For this review, take the finished solid that the model builds, in its own axes (mm). A direction names the side the tool comes from. Coordinates: 2 decimals unless noted, no trailing zeros. Loops run counter-clockwise (first coordinate to the right, second up) from the corner with the lowest first, then second, coordinate; pieces in that order, holes last. Notation, with made-up numbers: (-14.5, -29) -> (-9.5, -29) arc R6 ccw to (-9.5, -25) -> close; hole circle Ø2 at (32.25, 19.5). An arc over 180 degrees is marked (long way). One line per item, written item: value.
from build123d import *

# Parameters (mm, degrees)
F1_DEPTH  = 44.45
F9_DEPTH  = 9.525
F10_DEPTH = 9.525
F12_DEPTH = 2.38125
F13_R     = 11.7475
F13_R_2   = 10.7315
F14_DEPTH = 7.9375
F15_DEPTH = 10.31875


with BuildPart() as f1:
    # F0 (on Top) → F1 (new body)
    with BuildSketch(Plane.XY):
        with BuildLine():
            ThreePointArc((-4.572, 0), (0, 4.572), (4.572, 0))
            Line((4.572, 0), (7.747, 0))
            ThreePointArc((7.747, 0), (5.951410253, 4.9595085442), (1.397, 7.62))
            ThreePointArc((1.397, 7.62), (0, 7.747), (-1.397, 7.62))
            ThreePointArc((-1.397, 7.62), (-5.951410253, 4.9595085442), (-7.747, 0))
            Line((-7.747, 0), (-4.572, 0))
        make_face()
        with BuildLine():
            ThreePointArc((-1.397, 7.62), (0, 7.747), (1.397, 7.62))
            Line((1.397, 7.62), (1.397, 19.3802))
            ThreePointArc((1.397, 19.3802), (0, 19.1615406713), (-1.397, 19.3802))
            Line((-1.397, 19.3802), (-1.397, 7.62))
        make_face()
        with BuildLine():
            ThreePointArc((-1.397, 19.3802), (0, 19.1615406713), (1.397, 19.3802))
            ThreePointArc((1.397, 19.3802), (3.6939320514, 21.0394638349), (4.572, 23.7335406713))
            ThreePointArc((4.572, 23.7335406713), (-2.6940768363, 27.4274727226), (-1.397, 19.3802))
        make_face()
    extrude(amount=F1_DEPTH)

    # F6 (on offset) → F9 (cut)
    with BuildSketch(Plane.XY.offset(28.575)):
        with BuildLine():
            ThreePointArc((4.1557772601, 1.7640375299), (0, -1.016), (-4.1557772601, 1.7640375299))
            Line((-4.1557772601, 1.7640375299), (-7.6070004234, 1.7640375299))
            ThreePointArc((-7.6070004234, 1.7640375299), (0, -4.318), (7.6070004234, 1.7640375299))
            Line((7.6070004234, 1.7640375299), (4.1557772601, 1.7640375299))
        make_face()
        with BuildLine():
            ThreePointArc((-4.1557772601, 1.7640375299), (-0.8747878771, 7.8904367738), (4.4961791045, 3.4801791045))
            ThreePointArc((4.4961791045, 3.4801791045), (4.4102576693, 2.6053912274), (4.1557772601, 1.7640375299))
            Line((4.1557772601, 1.7640375299), (7.6070004234, 1.7640375299))
            ThreePointArc((7.6070004234, 1.7640375299), (7.750237064, 2.6168003938), (7.7981791045, 3.4801791045))
            ThreePointArc((7.7981791045, 3.4801791045), (-0.8633787106, 11.2304161684), (-7.6070004234, 1.7640375299))
            Line((-7.6070004234, 1.7640375299), (-4.1557772601, 1.7640375299))
        make_face()
        with BuildLine():
            ThreePointArc((7.6070004234, 1.7640375299), (0, -4.318), (-7.6070004234, 1.7640375299))
            Line((-7.6070004234, 1.7640375299), (-8.4216929972, 1.7640375299))
            Line((-8.4216929972, 1.7640375299), (-8.4216929972, -6.3198274001))
            Line((-8.4216929972, -6.3198274001), (11.7628639564, -6.3198274001))
            Line((11.7628639564, -6.3198274001), (11.7628639564, 1.7640375299))
            Line((11.7628639564, 1.7640375299), (7.6070004234, 1.7640375299))
        make_face()
    extrude(amount=F9_DEPTH, mode=Mode.SUBTRACT)

    # F8 (on offset) → F10 (cut)
    with BuildSketch(Plane.XY.offset(15.875)):
        with BuildLine():
            ThreePointArc((4.179462045, 1.8225532258), (0, -1.016), (-4.179462045, 1.8225532258))
            Line((-4.179462045, 1.8225532258), (-7.6199654718, 1.8225532258))
            ThreePointArc((-7.6199654718, 1.8225532258), (0, -4.318), (7.6199654718, 1.8225532258))
            Line((7.6199654718, 1.8225532258), (4.179462045, 1.8225532258))
        make_face()
        with BuildLine():
            ThreePointArc((-4.179462045, 1.8225532258), (-0.8438058499, 7.8964692022), (4.4961791045, 3.4801791045))
            ThreePointArc((4.4961791045, 3.4801791045), (4.4162900977, 2.6363732546), (4.179462045, 1.8225532258))
            Line((4.179462045, 1.8225532258), (7.6199654718, 1.8225532258))
            ThreePointArc((7.6199654718, 1.8225532258), (7.7534976902, 2.6465899292), (7.7981791045, 3.4801791045))
            ThreePointArc((7.7981791045, 3.4801791045), (-0.8335891753, 11.2336767947), (-7.6199654718, 1.8225532258))
            Line((-7.6199654718, 1.8225532258), (-4.179462045, 1.8225532258))
        make_face()
        with BuildLine():
            ThreePointArc((7.6199654718, 1.8225532258), (0, -4.318), (-7.6199654718, 1.8225532258))
            Line((-7.6199654718, 1.8225532258), (-8.5849482566, 1.8225532258))
            Line((-8.5849482566, 1.8225532258), (-8.5849482566, -5.9901881032))
            Line((-8.5849482566, -5.9901881032), (8.4006469697, -5.9901881032))
            Line((8.4006469697, -5.9901881032), (8.4006469697, 1.8225532258))
            Line((8.4006469697, 1.8225532258), (7.6199654718, 1.8225532258))
        make_face()
    extrude(amount=-F10_DEPTH, mode=Mode.SUBTRACT)

    # F11 (on face) → F12 (join)
    with BuildSketch(Plane.XY.offset(44.45)):
        with BuildLine():
            ThreePointArc((-1.397, 11.6641393703), (-7.7971949684, -8.7867802337), (11.7475, 0))
            ThreePointArc((11.7475, 0), (8.7867802337, 7.7971949684), (1.397, 11.6641393703))
            Line((1.397, 11.6641393703), (1.397, 7.62))
            ThreePointArc((1.397, 7.62), (5.951410253, 4.9595085442), (7.747, 0))
            Line((7.747, 0), (4.572, 0))
            ThreePointArc((4.572, 0), (0, -4.572), (-4.572, 0))
            Line((-4.572, 0), (-7.747, 0))
            ThreePointArc((-7.747, 0), (-5.951410253, 4.9595085442), (-1.397, 7.62))
            Line((-1.397, 7.62), (-1.397, 11.6641393703))
        make_face()
        with BuildLine():
            Line((1.397, 7.62), (1.397, 11.6641393703))
            ThreePointArc((1.397, 11.6641393703), (0, 11.7475), (-1.397, 11.6641393703))
            Line((-1.397, 11.6641393703), (-1.397, 7.62))
            ThreePointArc((-1.397, 7.62), (-5.951410253, 4.9595085442), (-7.747, 0))
            Line((-7.747, 0), (-4.572, 0))
            ThreePointArc((-4.572, 0), (0, 4.572), (4.572, 0))
            Line((4.572, 0), (7.747, 0))
            ThreePointArc((7.747, 0), (5.951410253, 4.9595085442), (1.397, 7.62))
        make_face()
    extrude(amount=F12_DEPTH)

    # F13 (on face) → F14 (join)
    with BuildSketch(Plane.XY.offset(46.83125)):
        Circle(F13_R)
        Circle(F13_R_2, mode=Mode.SUBTRACT)
    extrude(amount=F14_DEPTH)

    # F15 (add, through all): a face of the model
    f15_faces = [f1.faces().sort_by_distance(p)[0] for p in [
        (0, 21.7334038121, 44.45),
    ]]
    extrude(f15_faces, amount=F15_DEPTH)


solid = f1.part
1. The part is to be moulded in two halves that separate along Z. For faces 6 (the cylindrical face through (-4.23, 5, 11.18)), 7 (the flat face through (-6, 0, 41)), 8 (the flat face through (-1, 14, 0)), say which applies: pulls with the +Z half, pulls with the -Z half, needs draft (parallel to the pull), parting line crosses it, or undercut.
Return value:
face 6: undercut
face 7: needs draft
face 8: pulls with the -Z half
2. Insertion check: pin 1 Ø10.5 at (x, y) = (0, 0) entering from +Z; pin 2 Ø2.5 at (x, z) = (5.5, 39.5) entering from -Y; pin 3 Ø4 at (y, z) = (5, 18.5) entering from -X. Each pin has a flat end and moves straight along its axis. Give the tip position at first contact, or say it passes through.
Return value:
pin 1: stops at z = 46.83
pin 2: stops at y = 0
pin 3: stops at x = -7.14
3. Take a section at C-C, the plane z = 25. Give the boundary of the cut face in (x, y).
Return value:
outline: (-7.75, 0) -> (-4.57, 0) arc R4.57 cw to (4.57, 0) -> (7.75, 0) arc R7.75 ccw to (1.4, 7.62) -> (1.4, 19.38) arc R4.57 ccw (long way) to (-1.4, 19.38) -> (-1.4, 7.62) arc R7.75 ccw to start
4. Take a section at A-A, the plane x = 0. Give the number of separate pieces and of enclosed holes in the cut face, and give its area (3 significant figures).
Return value:
separate pieces: 2
enclosed holes: 2
area: 1,210 mm2
5. Take a section at D-D, the plane x = -9. Give the boundary of the cut face in (y, z), and give its area (3 significant figures).
Return value:
outline: (-7.55, 44.45) -> (7.55, 44.45) -> (7.55, 54.77) -> (5.85, 54.77) -> (5.85, 46.83) -> (-5.85, 46.83) -> (-5.85, 54.77) -> (-7.55, 54.77) -> close
area: 63.0 mm2
6. For faces 1 (the cylindrical face through (10.236, 3.223, 50.744)), 2 (the flat face through (-6, 3, 6.35)), 3 (the cylindrical face through (-0.02, 7.976, 11.179)), 4 (the flat face through (6, 0, 3)), 5 (the flat face through (6, 3, 28.575)), list the 3-axis set-ups (+Z, -Z, +X, -X, +Y, -Y) from which the entire face can be reached by the end or side of a thin tool; tool diameter is ignored.
Return value:
face 1: +Z
face 2: -X
face 3: none
face 4: -Z, +X, -X, -Y
face 5: +X
7. To check wall thickness, follow probe 1 along Z at (x, y) = (-6.75, 2.5) (3 decimals); probe 2 along Y at (x, z) = (0, 52); probe 3 along Z at (x, y) = (3.75, 3.5). State the ranges of each line that lie inside material, in increasing order. Write a range as from..to.
Return value:
probe 1: z = 0..6.35, 15.875..28.575, 38.1..46.831
probe 2: y = -11.75..-10.73, 10.73..28.31
probe 3: z = 0..46.83
8. Take a section at B-B, the plane z = 33. Give the boundary of the cut face in (x, y), and give its area (3 significant figures).
Return value:
outline: (-4.19, 1.84) arc R4.57 cw to (4.19, 1.84) arc R4.5 ccw to (2.1, 7.46) arc R7.75 ccw to (1.4, 7.62) -> (1.4, 7.75) arc R4.5 ccw to (-1.4, 7.75) -> (-1.4, 7.62) arc R7.75 ccw to (-2.1, 7.46) arc R4.5 ccw to start; (-1.4, 11.15) arc R7.8 cw to (1.4, 11.15) -> (1.4, 19.38) arc R4.57 ccw (long way) to (-1.4, 19.38) -> close
area: 118 mm2
